```python
from build123d import *

# Parameters (mm, degrees)
SWEEP1_PROFILE_R = 12.7
SHELL2_T         = -3.175


with BuildPart() as part:
    # Sweep1: sweep along a path in Sketch1
    with BuildLine(Plane.XY) as sweep1_path:
        Line((38.1, 786.13), (38.1, 25.4))
        ThreePointArc((38.1, 25.4), (30.660512242, 7.439487758), (12.7, 0))
        Line((12.7, 0), (0, 0))
    # Sweep1 profile (on start of the path) → Sweep1 (sweep)
    with BuildSketch(Plane(origin=(38.1, 786.13, 0), x_dir=(-1, 0, 0), z_dir=(0, -1, 0))):
        Circle(SWEEP1_PROFILE_R)
    sweep(path=sweep1_path.line)

    # Shell2
    shell2_openings = [part.faces().sort_by_distance(p)[0] for p in [
        (0, 0, 0),
        (38.1, 786.13, 0),
    ]]
    offset(amount=SHELL2_T, openings=shell2_openings, kind=Kind.INTERSECTION)


solid = part.part
```
Here's how the part is built. I have some questions about the finished solid (model axes, mm). A direction names the side the tool comes from. Coordinates: 2 decimals unless noted, no trailing zeros. Write each loop counter-clockwise with the first axis right and the second up, starting at its lowest first coordinate (ties: lowest second). Pieces come first, ordered by that corner, then holes. Notation, with made-up numbers: M -31.75,-14 L -17.75,-14 A22 ccw -17.75,-6 Z; hole C 62,28 d3. An arc over 180 degrees is marked long. Answer as CSV lines item,"result". Start each with the question number.
Q1. Will these pins go through, and if not, where does the flat tip stop? pin 1 Ø2 at (x, z) = (17, 5.5) entering from -Y; pin 2 Ø12 at (y, z) = (204, -0.5) entering from -X; pin 3 Ø2 at (x, z) = (16, -6) entering from +Y.
Q2. For faces 4 (the flat face through (48, 786.13, -2)), 5 (the cylindrical face through (6.26, -2.75, 12.4)), which set-ups out of +Z, -Z, +X, -X, +Y, -Y let a thin tool reach every point of the face, with its end or its side?
Q3. Suppose I cut it at B-B, the plane y = 53. List the corners of the cut face in (x, z) for me (3 decimals).
Q4. I need wall thicknesses on probe 1 along Y at (x, z) = (7.25, 0) (3 decimals); probe 2 along X at (y, z) = (420, 0) (3 decimals). Which ranges of each line are inside material? Lowest first, please. Write a range as [from, to].
Q5. Suppose I cut it at A-A, the plane z = 0. List the corners of the cut face in (x, y) for me (3 decimals), then the cut area to 3 significant figures.
Q6. If we mould it in two halves opening along Z, with no side actions, what happens to faces 1 (the flat face through (0, -9, -5)), 2 (the cylindrical face through (29.3, 400.44, 3.65)), 3 (the cylindrical face through (48.2, 400.4, 7.7))? For each: pulls with the +Z half, pulls with the -Z half, needs draft (parallel to the pull), parting line crosses it, or undercut.
Entries:
1,pin 1,"stops at y = -11.64"
1,pin 2,"stops at x = 25.4"
1,pin 3,"stops at y = 12.15"
2,face 4,"+Z, -Z, +X, -X, +Y"
2,face 5,"-X"
3,outline,"C 38.1,0 d25.4; hole C 38.1,0 d19.05"
4,probe 1,"y = [-12.7, -9.525], [9.525, 12.7]"
4,probe 2,"x = [25.4, 28.575], [47.625, 50.8]"
5,outline,"M 0,-12.7 L 12.7,-12.7 A38.1 ccw 50.8,25.4 L 50.8,786.13 L 47.625,786.13 L 47.625,25.4 A34.925 cw 12.7,-9.525 L 0,-9.525 Z; M 0,9.525 L 12.7,9.525 A15.875 ccw 28.575,25.4 L 28.575,786.13 L 25.4,786.13 L 25.4,25.4 A12.7 cw 12.7,12.7 L 0,12.7 Z"
5,area,"5,160 mm²"
6,face 1,"needs draft"
6,face 2,"undercut"
6,face 3,"parting line crosses it"
